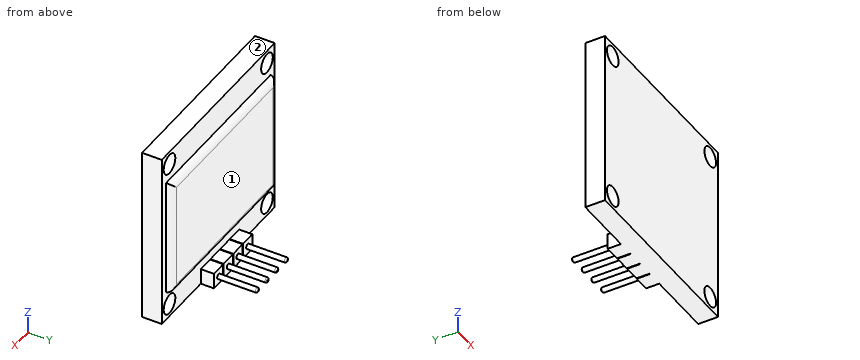
```python
from build123d import *

# Parameters (mm, degrees)
SKETCH1_W           = 29.18
SKETCH1_H           = 27.1
BOSS_EXTRUDE1_DEPTH = 3
SKETCH2_W           = 27
SKETCH2_H           = 18
BOSS_EXTRUDE2_DEPTH = 1
FILLET1_R           = 1
SKETCH3_R           = 1.5
CUT_EXTRUDE1_DEPTH  = 21.136300554
SKETCH4_W           = 2.4
SKETCH4_H           = 2.4
BOSS_EXTRUDE3_DEPTH = 2
SKETCH5_R           = 0.375
BOSS_EXTRUDE4_DEPTH = 6
FILLET2_R           = 0.2


with BuildPart() as part:
    # Sketch1 → Boss-Extrude1 (new body)
    with BuildSketch(Plane(origin=(0, 0, 0), x_dir=(1, 0, 0), z_dir=(0, 1, 0))):
        Rectangle(SKETCH1_W, SKETCH1_H)
    extrude(amount=BOSS_EXTRUDE1_DEPTH)

    # Sketch2 → Boss-Extrude2 (add)
    with BuildSketch(Plane(origin=(0, 3, 0), x_dir=(1, 0, 0), z_dir=(0, 1, 0))):
        Rectangle(SKETCH2_W, SKETCH2_H)
    extrude(amount=BOSS_EXTRUDE2_DEPTH)

    # Fillet1
    fillet1_edges = [part.edges().sort_by_distance(p)[0] for p in [
        (0, 4, -9),
        (13.5, 4, 0),
        (0, 4, 9),
        (-13.5, 4, 0),
    ]]
    fillet(fillet1_edges, radius=FILLET1_R - 0.0001)  # a hair under: the kernel refuses the full size

    # Sketch3 → Cut-Extrude1 (cut, through all)
    with BuildSketch(Plane(origin=(0, 3, 0), x_dir=(1, 0, 0), z_dir=(0, 1, 0))):
        with Locations(Location((-12.59, 11.55, 0), (0, 0, 270))):
            Circle(SKETCH3_R)
        with Locations(Location((12.59, 11.55, 0), (0, 0, 270))):
            Circle(SKETCH3_R)
        with Locations(Location((12.59, -11.55, 0), (0, 0, 90))):
            Circle(SKETCH3_R)
        with Locations(Location((-12.59, -11.55, 0), (0, 0, 90))):
            Circle(SKETCH3_R)
    extrude(amount=-CUT_EXTRUDE1_DEPTH, mode=Mode.SUBTRACT)

    # Sketch4 → Boss-Extrude3 (add)
    with BuildSketch(Plane(origin=(0, 3, 0), x_dir=(1, 0, 0), z_dir=(0, 1, 0))):
        with Locations((-4.19, 12.35)):
            Rectangle(SKETCH4_W, SKETCH4_H)
        with Locations((-1.69, 12.35)):
            Rectangle(SKETCH4_W, SKETCH4_H)
        with Locations((0.81, 12.35)):
            Rectangle(SKETCH4_W, SKETCH4_H)
        with Locations((3.31, 12.35)):
            Rectangle(SKETCH4_W, SKETCH4_H)
    extrude(amount=BOSS_EXTRUDE3_DEPTH)

    # Sketch5 → Boss-Extrude4 (add)
    with BuildSketch(Plane(origin=(0, 5, 0), x_dir=(1, 0, 0), z_dir=(0, 1, 0))):
        with Locations(Location((-4.19, 12.35, 0), (0, 0, 90))):
            Circle(SKETCH5_R)
        with Locations(Location((-1.69, 12.35, 0), (0, 0, 90))):
            Circle(SKETCH5_R)
        with Locations(Location((0.81, 12.35, 0), (0, 0, 90))):
            Circle(SKETCH5_R)
        with Locations(Location((3.31, 12.35, 0), (0, 0, 90))):
            Circle(SKETCH5_R)
    extrude(amount=BOSS_EXTRUDE4_DEPTH)

    # Fillet2
    fillet2_edges = [part.edges().sort_by_distance(p)[0] for p in [
        (-4.19, 11, -11.975),
        (-1.69, 11, -11.975),
        (0.81, 11, -11.975),
        (3.31, 11, -11.975),
    ]]
    fillet(fillet2_edges, radius=FILLET2_R)


solid = part.part
```
Model file for the job. Use its own axes, mm. Face numbers are marked on the shaded views. A direction names the side the tool comes from. Coordinates: 2 decimals unless noted, no trailing zeros. Loops run counter-clockwise (first coordinate to the right, second up) from the corner with the lowest first, then second, coordinate; pieces in that order, holes last. Notation, with made-up numbers: (-33, 21) -> (26, 21) arc R20 cw to (26, 41) -> close; hole circle Ø4 at (27.25, 81). An arc over 180 degrees is marked (long way). Answer as a JSON object with one key per item and string values.
Q1. Cut at A-A (z = -11.55). List the corners of the cut face in (x, y), and give its area (3 significant figures).
Report:
{"outline": "(-14.59, 0) -> (-14.09, 0) -> (-14.09, 3) -> (-14.59, 3) -> close; (-11.09, 0) -> (11.09, 0) -> (11.09, 3) -> (4.51, 3) -> (4.51, 5) -> (2.11, 5) -> (2.11, 3) -> (2.01, 3) -> (2.01, 5) -> (-0.39, 5) -> (-0.39, 3) -> (-0.49, 3) -> (-0.49, 5) -> (-2.89, 5) -> (-2.89, 3) -> (-2.99, 3) -> (-2.99, 5) -> (-5.39, 5) -> (-5.39, 3) -> (-11.09, 3) -> close; (14.09, 0) -> (14.59, 0) -> (14.59, 3) -> (14.09, 3) -> close", "area": "88.7 mm2"}
Q2. Cut at B-B (y = 3.5). List the corners of the cut face in (x, z), and give its area (3 significant figures).
Report:
{"outline": "(-13.37, -8.87) -> (13.37, -8.87) -> (13.37, 8.87) -> (-13.37, 8.87) -> close; (-5.39, -13.55) -> (-2.99, -13.55) -> (-2.99, -11.15) -> (-5.39, -11.15) -> close; (-2.89, -13.55) -> (-0.49, -13.55) -> (-0.49, -11.15) -> (-2.89, -11.15) -> close; (-0.39, -13.55) -> (2.01, -13.55) -> (2.01, -11.15) -> (-0.39, -11.15) -> close; (2.11, -13.55) -> (4.51, -13.55) -> (4.51, -11.15) -> (2.11, -11.15) -> close", "area": "497 mm2"}
Q3. Probe probe 1 along X at (y, z) = (2, 11.55); probe 2 along Y at (x, z) = (3.5, -6.5); probe 3 along Z at (x, y) = (0.75, 4.5). List the from-to ranges inside material, lowest first.
Report:
{"probe 1": "x = -14.59 to -14.09, -11.09 to 11.09, 14.09 to 14.59", "probe 2": "y = 0 to 4", "probe 3": "z = -13.55 to -11.15"}
Q4. 3-axis set-ups, long thin cutter, end or side, ignore diameter. For the marked faces 1 and 2: which of +Z, -Z, +X, -X, +Y, -Y reach the whole face in a straight line?
Report:
{"face 1": "+Z, +X, -X, +Y", "face 2": "+Z, +X, -X, +Y, -Y"}
Q5. Flat gauge pins, fed straight in: P1, Ø1.6, axis at x = 3, y = 4, coming from the +Z side; P2, Ø6, axis at x = 6, y = 9, coming from the +Z side (3 decimals); P3, Ø0.6, axis at y = 3.5, z = -12, coming from the +X side. Where does each tip first touch, or does it go through?
Report:
{"P1": "stops at z = 8.98", "P2": "stops at z = -11.975", "P3": "stops at x = 4.51"}
